```python
from build123d import *

# Parameters (mm, degrees)
F2_SIZE2  = 1.99999
F2_SIZE   = 1.99999
F5_R      = 5.75
F6_DEPTH  = 25
F7_R      = 5.75
F8_DEPTH  = 25
F10_DEPTH = 25


# Not quite as in the source:
# - a fillet or chamfer is up to 0.001 mm smaller than in the source, because OpenCascade refuses the exact size


with BuildPart() as f1:
    # F0 (on Front) → F1 (revolve)
    with BuildSketch(Plane.XZ):
        with BuildLine():
            Line((8.64674, 2), (7.25, 2))
            Line((7.25, 2), (7.25, 41))
            Line((7.25, 41), (5.75, 41))
            Line((5.75, 41), (5.75, 40))
            Line((5.75, 40), (4.75, 40))
            Line((4.75, 40), (4.75, 39))
            ThreePointArc((4.75, 39), (5.4571067812, 38.7071067812), (5.75, 38))
            Line((5.75, 38), (5.75, 4.9999998882))
            ThreePointArc((5.75, 4.9999998882), (5.4571067812, 4.2928931071), (4.75, 3.9999998882))
            Line((4.75, 3.9999998882), (4.75, 2.9999998882))
            Line((4.75, 2.9999998882), (5.75, 2.9999998882))
            Line((5.75, 2.9999998882), (5.75, 0))
            Line((5.75, 0), (8.64674, 0))
            Line((8.64674, 0), (8.64674, 2))
        make_face()
    revolve(axis=Axis((0, 0, 27.7979653329), (0, 0, 1)))

    # F2 (size 2 and 2 in the source; OpenCascade refuses exactly that, so slightly less here)
    f2_edges = [f1.edges().sort_by_distance(p)[0] for p in [
        (-8.64674, 0, 0),
    ]]
    chamfer(f2_edges, length=F2_SIZE, length2=F2_SIZE2)

    # F3 (on Front) → F4 (revolve)
    with BuildSketch(Plane.XZ):
        with BuildLine():
            Line((0, 55), (0, 41))
            Line((0, 41), (0, 40))
            Line((0, 40), (5.75, 40))
            Line((5.75, 40), (5.75, 46))
            add(Edge.make_bspline(
                [(0, 55), (0.1440579667, 54.8954034218), (0.4017096448, 54.5348723025), (0.9570213075, 53.3087861702), (1.7966593586, 47.7287211885), (2.1990543329, 44.2884011591), (2.9678127556, 43.2712194265), (4.3524509198, 44.1285353141), (5.1923480343, 45.0871969322), (5.5351351682, 45.7667505271), (5.75, 46)],
                knots=[0, 0, 0, 0, 0.0706016145, 0.1776436842, 0.4082606642, 0.5899939047, 0.6786962714, 0.7910306665, 0.9027344001, 1, 1, 1, 1], degree=3))
        make_face()
    revolve(axis=Axis((0, 0, 2), (0, 0, 1)))

    # F5 (on face) → F6 (cut)
    with BuildSketch(Plane(origin=(0, 0, 40), x_dir=(1, 0, 0), z_dir=(0, 0, -1))):
        Circle(F5_R)
    extrude(amount=F6_DEPTH, mode=Mode.SUBTRACT)

    # F7 (on face) → F8 (cut)
    with BuildSketch(Plane(origin=(0, 0, 2.9999998882), x_dir=(1, 0, 0), z_dir=(0, 0, -1))):
        Circle(F7_R)
    extrude(amount=-F8_DEPTH, mode=Mode.SUBTRACT)

    # F9 (on face) → F10 (cut)
    with BuildSketch(Plane(origin=(0, 0, 40), x_dir=(1, 0, 0), z_dir=(0, 0, -1))):
        with BuildLine():
            ThreePointArc((3.5453054724, 1.222010273), (3.75, 0), (3.5453054724, -1.222010273))
            Line((3.5453054724, -1.222010273), (4.7270739632, -1.6293470307))
            ThreePointArc((4.7270739632, -1.6293470307), (5, 0), (4.7270739632, 1.6293470307))
            Line((4.7270739632, 1.6293470307), (3.5453054724, 1.222010273))
        make_face()
        with BuildLine():
            Line((3.1658679099, 2.0099204903), (4.2211572131, 2.6798939871))
            ThreePointArc((4.2211572131, 2.6798939871), (3.1174490093, 3.9091574123), (1.6734076042, 4.7116565017))
            Line((1.6734076042, 4.7116565017), (1.2550557032, 3.5337423763))
            ThreePointArc((1.2550557032, 3.5337423763), (2.338086757, 2.9318680593), (3.1658679099, 2.0099204903))
        make_face()
        with BuildLine():
            Line((0.4024672392, 3.7283401295), (0.5366229857, 4.9711201727))
            ThreePointArc((0.5366229857, 4.9711201727), (-1.1126046698, 4.8746395609), (-2.640368812, 4.2459925267))
            Line((-2.640368812, 4.2459925267), (-1.980276609, 3.184494395))
            ThreePointArc((-1.980276609, 3.184494395), (-0.8344535023, 3.6559796707), (0.4024672392, 3.7283401295))
        make_face()
        with BuildLine():
            Line((-2.6639994714, 2.6392436069), (-3.5519992951, 3.5189914759))
            ThreePointArc((-3.5519992951, 3.5189914759), (-4.5048443395, 2.1694186956), (-4.9658936591, 0.5830095766))
            Line((-4.9658936591, 0.5830095766), (-3.7244202443, 0.4372571824))
            ThreePointArc((-3.7244202443, 0.4372571824), (-3.3786332546, 1.6270640217), (-2.6639994714, 2.6392436069))
        make_face()
        with BuildLine():
            Line((-3.7244202443, -0.4372571824), (-4.9658936591, -0.5830095766))
            ThreePointArc((-4.9658936591, -0.5830095766), (-4.5048443395, -2.1694186956), (-3.5519992951, -3.5189914759))
            Line((-3.5519992951, -3.5189914759), (-2.6639994714, -2.6392436069))
            ThreePointArc((-2.6639994714, -2.6392436069), (-3.3786332546, -1.6270640217), (-3.7244202443, -0.4372571824))
        make_face()
        with BuildLine():
            Line((-1.980276609, -3.184494395), (-2.640368812, -4.2459925267))
            ThreePointArc((-2.640368812, -4.2459925267), (-1.1126046698, -4.8746395609), (0.5366229857, -4.9711201727))
            Line((0.5366229857, -4.9711201727), (0.4024672392, -3.7283401295))
            ThreePointArc((0.4024672392, -3.7283401295), (-0.8344535023, -3.6559796707), (-1.980276609, -3.184494395))
        make_face()
        with BuildLine():
            Line((1.2550557032, -3.5337423763), (1.6734076042, -4.7116565017))
            ThreePointArc((1.6734076042, -4.7116565017), (3.1174490093, -3.9091574123), (4.2211572131, -2.6798939871))
            Line((4.2211572131, -2.6798939871), (3.1658679099, -2.0099204903))
            ThreePointArc((3.1658679099, -2.0099204903), (2.338086757, -2.9318680593), (1.2550557032, -3.5337423763))
        make_face()
    extrude(amount=-F10_DEPTH, mode=Mode.SUBTRACT)


solid = f1.part
```
Work out the finished part from the listing and answer in its coordinate system (mm). A direction names the side the tool comes from. Coordinates: 2 decimals unless noted, no trailing zeros. Order: outer loops, then holes, each group sorted by start corner. A loop starts at its lowest first (then second) coordinate and runs counter-clockwise, first axis right, second up. Notation, with made-up numbers: M 88.25,-27.5 L 128.25,-27.5 A24 ccw 128.25,1.5 Z; hole C 21,45 d1. An arc over 180 degrees is marked long. Use CSV: the item, a comma, the result in double quotes.
1) Consider line 1 (Y direction, x = 0, z = 19.5); line 2 (X direction, y = 3, z = 40.5); line 3 (X direction, y = -0.25, z = 38). Determine where each line is inside the solid, lowest interval first. Write a range as [from, to].
Worked out:
line 1,"y = [-7.25, -5.75], [5.75, 7.25]"
line 2,"x = [-6.6, -4], [-3.03, 2.25], [4, 6.6]"
line 3,"x = [-7.25, -5.74], [5.74, 7.25]"
2) Section A-A on z = 13 is taken. Write down the section's boundary in (x, y).
Worked out:
outline,"C 0,0 d14.5; hole C 0,0 d11.5"
3) Determine the mould class of faces 1 (the face through (4, 4.5, 0)), 2 (the face through (-0.75, 5.7, 43.54)), 3 (the face through (3.75, -0.02, 41.87)) for opening direction X: released by +X, released by -X, zero draft, split by the parting line, or undercut.
Worked out:
face 1,"zero draft"
face 2,"split by the parting line"
face 3,"undercut"
4) For faces 4 (the face through (1.46, 4.11, 41.87)), 5 (the face through (0, 0, 40)), 6 (the face through (-5, -6, 2)), determine the directions among +Z, -Z, +X, -X, +Y, -Y from which every point of the face is accessible in a straight line to the end or side of a thin tool.
Worked out:
face 4,"+Z, -Z"
face 5,"-Z"
face 6,"+Z"
5) Flat-ended cylindrical pins translate along their axes: pin 1 Ø10 at (y, z) = (-2.5, 47) entering from -X; pin 2 Ø5 at (x, z) = (-0.5, 12) entering from -Y; pin 3 Ø1 at (x, y) = (5, 2) entering from +Z; pin 4 Ø10 at (x, y) = (-0.5, -1) entering from -Z. Find the tip coordinate at first contact, or state that the pin passes through.
Worked out:
pin 1,"stops at x = -5.75"
pin 2,"stops at y = -7.25"
pin 3,"stops at z = 46"
pin 4,"stops at z = 0"
